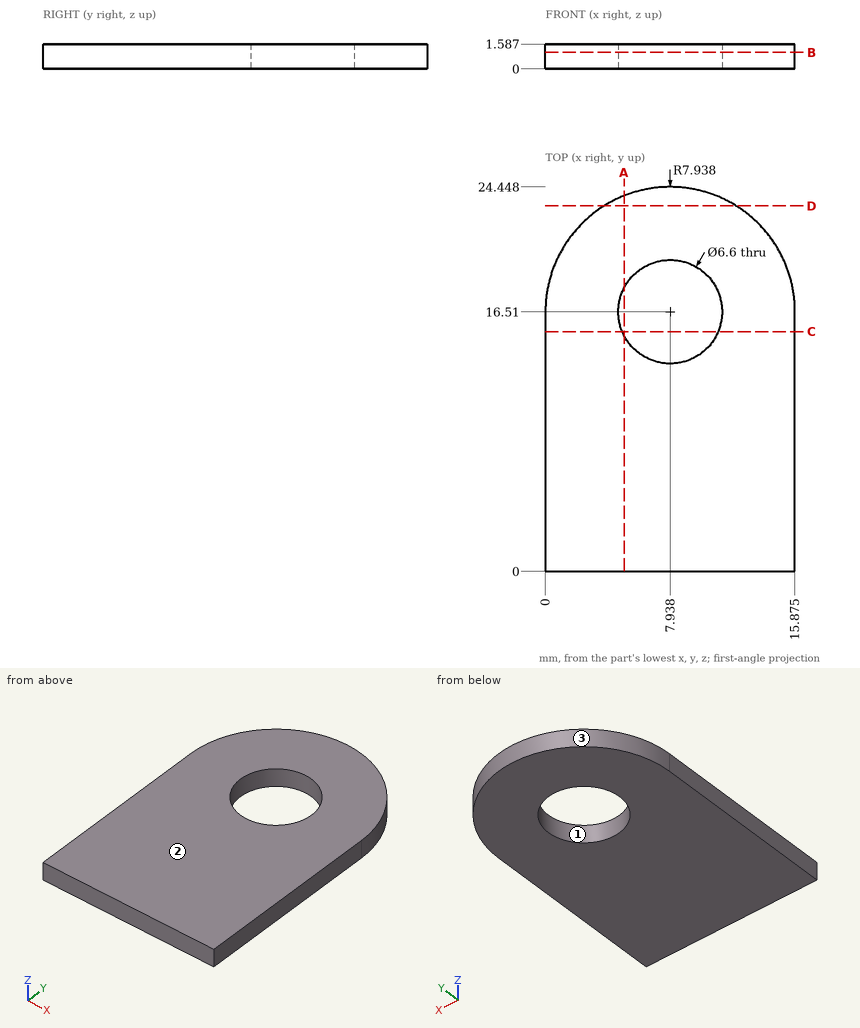
Here's the drawing with two shaded views (mm, measured from the low corner). I have some questions. Give positions to 0.01 mm unless a question says otherwise; leave off trailing zeros. Loops run counter-clockwise (first coordinate to the right, second up) from the corner with the lowest first, then second, coordinate; pieces in that order, holes last. Notation, with made-up numbers: M 14,3.25 L 33,3.25 A21 cw 33,35.25 Z; hole C 41,59 d8. An arc over 180 degrees is marked long. One line per item, written item: value.
(1) Suppose I cut it at B-B on z = 1.05. List the corners of the cut face in (x, y) for me (1 decimal).
Returned:
outline: M 0,0 L 15.9,0 L 15.9,16.5 A7.9 ccw 0,16.5 Z; hole C 7.9,16.5 d6.6
(2) Will this pin go through, and if not, where does the flat tip stop? pin 1 (1.5 mm diameter, centred on x = 9.5, y = 8.5, fed in from -Z).
Returned:
pin 1: z = 0
(3) Suppose I cut it at A-A on x = 5. List the corners of the cut face in (y, z) for me.
Returned:
outline: M 0,0 L 15.01,0 L 15.01,1.59 L 0,1.59 Z; M 18.01,0 L 23.88,0 L 23.88,1.59 L 18.01,1.59 Z
(4) We'd pull the mould along Y, two halves only. Please class the marked faces 1, 2 and 3: released by +Y, released by -Y, zero draft, split by the parting line, or undercut.
Returned:
face 1: undercut
face 2: zero draft
face 3: released by +Y
(5) I need wall thicknesses on line 1 (X direction, y = 14.5, z = 0.2) (1 decimal); line 2 (X direction, y = 13.5, z = 1.5) (1 decimal); line 3 (Y direction, x = 5.25, z = 0.9) (1 decimal). Which ranges of each line are inside material? Lowest first, please.
Returned:
line 1: 0 to 5.3, 10.6 to 15.9
line 2: 0 to 6.6, 9.3 to 15.9
line 3: 0 to 14.6, 18.4 to 24
(6) Suppose I cut it at D-D on y = 23.25. List the corners of the cut face in (x, z) for me (1 decimal).
Returned:
outline: M 3.7,0 L 12.1,0 L 12.1,1.6 L 3.7,1.6 Z
(7) Suppose I cut it at C-C on y = 15.25. List the corners of the cut face in (x, z) for me (1 decimal).
Returned:
outline: M 0,0 L 4.9,0 L 4.9,1.6 L 0,1.6 Z; M 11,0 L 15.9,0 L 15.9,1.6 L 11,1.6 Z
